Source: CAD feature listing. Evaluate the final solid. Frame: model axes, mm. A direction names the side the tool comes from. Give positions to 0.01 mm unless a question says otherwise; leave off trailing zeros. Order: outer loops, then holes, each group sorted by start corner. A loop starts at its lowest first (then second) coordinate and runs counter-clockwise, first axis right, second up.
```python
from build123d import *

# Parameters (mm, degrees)
SKETCH5_W               = 1.587499994
SKETCH5_H               = 55.780081988
CUT_EXTRUDE5_DEPTH      = 80.097038204
CUT_EXTRUDE5_DEPTH_BACK = 80.097038204
SKETCH7_R               = 1.5875
CUT_EXTRUDE6_DEPTH      = 80.097038326
CUT_EXTRUDE6_DEPTH_BACK = 80.097038326
SKETCH6_R               = 1.5875
SKETCH10_R              = 7.9375
BOSS_EXTRUDE1_DEPTH     = 30.380081988


with BuildPart() as part:
    # Sketch5 → Revolve2 (revolve)
    with BuildSketch(Plane(origin=(0, 0, 0), x_dir=(1, 0, 0), z_dir=(0, 1, 0)), mode=Mode.PRIVATE) as revolve2_sk:
        with Locations((8.731249997, -50.051540994)):
            Rectangle(SKETCH5_W, SKETCH5_H)
    revolve(revolve2_sk.sketch.rotate(Axis((0, 0, 0), (0, 0, 1)), 180), axis=Axis((0, 0, 0), (0, 0, 1)))

    # Sketch7 → Cut-Extrude5 (cut, two sides: drawn at the far end of the back side and taken through both)
    with BuildSketch(Plane(origin=(0, 0, 0), x_dir=(0, 0, -1), z_dir=(1, 0, 0)).offset(-CUT_EXTRUDE5_DEPTH_BACK)):
        with Locations((-39.195999993, 0)):
            Circle(SKETCH7_R)
    extrude(amount=CUT_EXTRUDE5_DEPTH + CUT_EXTRUDE5_DEPTH_BACK, mode=Mode.SUBTRACT)

    # Sketch6 → Cut-Extrude6 (cut, two sides: drawn at the far end of the back side and taken through both)
    with BuildSketch(Plane(origin=(0, 0, 0), x_dir=(1, 0, 0), z_dir=(0, 1, 0)).offset(-CUT_EXTRUDE6_DEPTH_BACK)):
        with Locations(Location((1e-09, -33.163499999, 0), (0, 0, 269.999999955))):
            Circle(SKETCH6_R)
    extrude(amount=CUT_EXTRUDE6_DEPTH + CUT_EXTRUDE6_DEPTH_BACK, mode=Mode.SUBTRACT)

    # Sketch10 → Boss-Extrude1 (add)
    with BuildSketch(Plane(origin=(0, 0, 47.5615), x_dir=(-1, 0, 0), z_dir=(0, 0, -1))):
        Circle(SKETCH10_R)
    extrude(amount=-BOSS_EXTRUDE1_DEPTH)


solid = part.part
```
1) Section query A-A, the plane x = 0. Return the cut outline in (y, z) (1 decimal), and give its area (3 significant figures).
Report:
outline: (-9.5, 22.2) - (-7.9, 22.2) - (-7.9, 31.6) - (-9.5, 31.6) - close; (-9.5, 34.8) - (-7.9, 34.8) - (-7.9, 47.6) - (7.9, 47.6) - (7.9, 34.8) - (9.5, 34.8) - (9.5, 77.9) - (-9.5, 77.9) - close; (7.9, 22.2) - (9.5, 22.2) - (9.5, 31.6) - (7.9, 31.6) - close
area: 649 mm2
2) Draft query along X for faces 3 (the cylindrical face through (-8.66, 0.07, 40.78)), 4 (the cylindrical face through (-4.4, 8.45, 49.66)), 5 (the flat face through (0, 0, 47.562)). Return one class per face: +X half, -X half, draft (parallel to the pull), parting line (faces both ways), or undercut.
Report:
face 3: draft
face 4: parting line
face 5: undercut
3) Section query D-D, the plane x = 6.5. Return the cut outline in (y, z), and give its area (3 significant figures).
Report:
outline: (-6.96, 22.16) - (-4.56, 22.16) - (-4.56, 47.56) - (4.56, 47.56) - (4.56, 22.16) - (6.96, 22.16) - (6.96, 77.94) - (-6.96, 77.94) - close
area: 545 mm2
4) Pin query (flat end, axial travel): pin 1 (2 mm diameter, centred on y = -2, z = 49, fed in from +X); pin 2 (6 mm diameter, centred on x = 5, z = 32, fed in from +Y); pin 3 (2 mm diameter, centred on x = -3.5, y = 1.5, fed in from -Z). Return the tip coordinate at first contact, or that it passes through.
Report:
pin 1: stops at x = 9.47
pin 2: stops at y = 9.31
pin 3: stops at z = 47.56
5) Material intervals for L1, parallel to Y at x = 0, z = 30.75 (1 decimal); L2, parallel to Z at x = 8.4, y = 0; L3, parallel to Z at x = 0, y = -9.1, sorted ascending.
Report:
L1: y = -9.5 to -7.9, 7.9 to 9.5
L2: z = 22.16 to 37.61, 40.78 to 77.94
L3: z = 22.16 to 31.58, 34.75 to 77.94
6) Section query B-B, the plane y = 0. Return the cut outline in (x, z) (1 decimal), and give its area (3 significant figures).
Report:
outline: (-9.5, 22.2) - (-7.9, 22.2) - (-7.9, 37.6) - (-9.5, 37.6) - close; (-9.5, 40.8) - (-7.9, 40.8) - (-7.9, 47.6) - (7.9, 47.6) - (7.9, 40.8) - (9.5, 40.8) - (9.5, 77.9) - (-9.5, 77.9) - close; (7.9, 22.2) - (9.5, 22.2) - (9.5, 37.6) - (7.9, 37.6) - close
area: 649 mm2
7) Reachability of faces 1 (the cylindrical face through (0.07, -8.663, 31.578)), 2 (the cylindrical face through (-7.332, 3.04, 34.684)) from +Z, -Z, +X, -X, +Y, -Y: full face, straight path, thin tool, end or side. Return the list, or none.
Report:
face 1: +Y, -Y
face 2: -Z
